Check sheet for the drawn part. Datum: minimum x, y, z corner. Units: mm. A direction names the side the tool comes from. Give positions to 0.01 mm unless a question says otherwise; leave off trailing zeros. Loops run counter-clockwise (first coordinate to the right, second up) from the corner with the lowest first, then second, coordinate; pieces in that order, holes last. Notation, with made-up numbers: (77, -34.75) - (85, -34.75) arc R34 cw to (85, -0.75) - close; hole circle Ø4 at (47, 40.25). An arc over 180 degrees is marked (long way). Use one line per item in the form item = value.
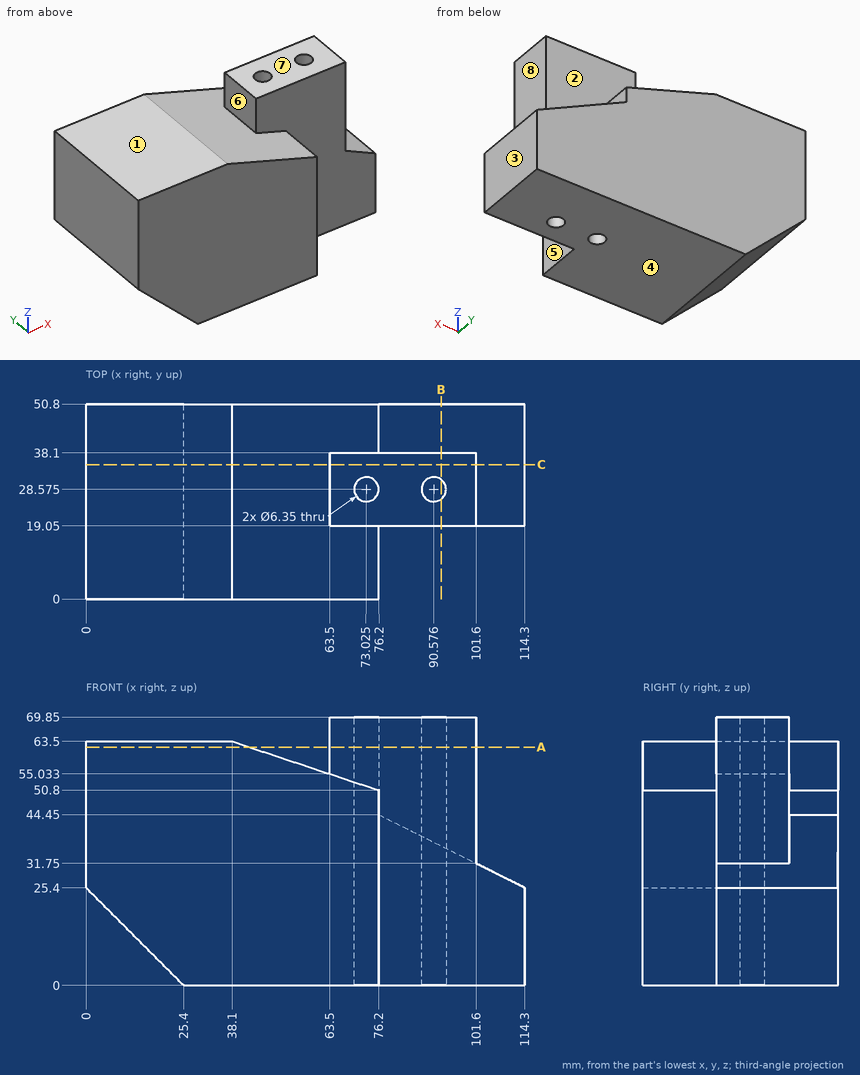
Item 1: Mould release check, pull along X, two halves, no side actions. Record for the marked faces 6, 7 and 8: released by +X, released by -X, zero draft, split by the parting line, or undercut.
Answer block:
face_6 = undercut
face_7 = zero draft
face_8 = released by +X
Item 2: Thickness scan on L1, parallel to Y at x = 90.5, z = 25; L2, parallel to X at y = 27, z = 11.5; L3, parallel to Y at x = 97, z = 38.5. Record the ranges inside material, lowest first.
Answer block:
L1 = 19.05 to 25.4, 31.75 to 50.8
L2 = 13.9 to 70.27, 75.78 to 87.82, 93.33 to 114.3
L3 = 19.05 to 38.1
Item 3: Access from +Z, -Z, +X, -X, +Y, -Y to the whole of each face (thin tool, end or side, straight path). Record for the marked faces 1, 2, 3, 4 and 5.
Answer block:
face_1 = +Z, -X, +Y, -Y
face_2 = +Z, +X, +Y
face_3 = +Z, -Z, +X, +Y, -Y
face_4 = -Z, +X, -X, +Y, -Y
face_5 = +Z, -Z, +X, -Y
Item 4: Section check C-C on y = 35. Record the boundary of the cut face in (x, z).
Answer block:
outline = (0, 25.4) - (25.4, 0) - (114.3, 0) - (114.3, 25.4) - (101.6, 31.75) - (101.6, 69.85) - (63.5, 69.85) - (63.5, 55.03) - (38.1, 63.5) - (0, 63.5) - close
Item 5: Section check B-B on x = 92.5. Record the boundary of the cut face in (y, z).
Answer block:
outline = (19.05, 0) - (26.05, 0) - (26.05, 69.85) - (19.05, 69.85) - close; (31.1, 0) - (50.8, 0) - (50.8, 36.3) - (38.1, 36.3) - (38.1, 69.85) - (31.1, 69.85) - close
Item 6: Section check A-A on z = 62. Give the number of separate pieces and of enclosed holes in the cut face, then the cut area to 3 significant figures.
Answer block:
separate_pieces = 2
enclosed_holes = 2
area = 2,830 mm2
Item 7: Gauge pin test, flat ends, axial feed: P1, Ø5.5, axis at x = 90.58, y = 28.58, coming from the -Z side; P2, Ø10, axis at x = 15.5, y = 16.5, coming from the +Z side; P3, Ø8, axis at x = 81, z = 33, coming from the -Y side; P4, Ø21, axis at y = 7.5, z = 19.5, coming from the +X side. Record the tip position at first contact, or that the pin passes through.
Answer block:
P1 = through
P2 = 63.5
P3 = 19.05
P4 = 76.2
